For this review, take the finished solid that the model builds, in its own axes (mm). Coordinates: 2 decimals unless noted, no trailing zeros. Loops run counter-clockwise (first coordinate to the right, second up) from the corner with the lowest first, then second, coordinate; pieces in that order, holes last. Notation, with made-up numbers: (73, -30) - (104, -30) arc R16 ccw to (104, -22) - close; hole circle Ø10 at (43.25, 86). An arc over 180 degrees is marked (long way). Use one line per item in the form item = value. Start each with the question number.
1. For pin 1 Ø2 at (x, y) = (18, 4.5) entering from +Z, flat-tipped, find the tip position at first contact; note if it passes through.
2. Add section A-A on x = 0. Give the boundary of the cut face in (y, z), and give its area (3 significant figures).
3. Add section B-B on z = 0. Give the boundary of the cut face in (x, y), and give its area (3 significant figures).
4. To check wall thickness, follow probe 1 along Z at (x, y) = (0, 1.75); probe 2 along Z at (x, y) = (7, 0.75); probe 3 along X at (y, z) = (2.75, -31.5). State the ranges of each line that lie inside material, in increasing order.
5. Add section D-D on x = -11.5. Give the boundary of the cut face in (y, z), and give its area (3 significant figures).
6. Add section C-C on y = 4.25. Give the boundary of the cut face in (x, z) (1 decimal), and give its area (3 significant figures).
7. Draft analysis for pull direction Z (two halves, no side actions). For faces 1 (the face through (0.414, 3.131, 21.586)), 2 (the face through (3.097, 3.131, -24.152)), 3 (the face through (0, 0, -22)), 4 (the face through (14.274, 3.131, -0.628)), state which applies: +Z half, -Z half, draft (parallel to the pull), parting line (faces both ways), or undercut.
Autodesk Inventor part; units mm, degrees
ref_plane "YZ Plane" through (0, 0, 0) normal (1, 0, 0) x (0, 1, 0)
ref_plane "XZ Plane" through (0, 0, 0) normal (0, 1, 0) x (-1, 0, 0)
ref_plane "XY Plane" through (0, 0, 0) normal (0, 0, 1) x (1, 0, 0)
sketch "Sketch1" plane through (0, 0, 0) normal (0, 1, 0) x (-1, 0, 0)
  circle A0 centre (0, 0) radius 15.24 construction
  circle A1 centre (0, -38.1) radius 22.86 construction
  circle A2 centre (0, 0) radius 14.2875
  circle A3 centre (0, -38.1) radius 14.2875
  line L0 (-14.9321, 3.048) -> (-22.3981, -33.528) construction
  line L1 (14.9321, 3.048) -> (22.3981, -33.528) construction
  arc A4 (-22.3981, -33.528) -> (22.3981, -33.528) centre (0, -38.1) ccw construction
  arc A5 (14.9321, 3.048) -> (-14.9321, 3.048) centre (0, 0) ccw construction
  line L2 (28.6198, -32.258) -> (21.1538, 4.318)
  arc A6 (21.1538, 4.318) -> (-21.1538, 4.318) centre (0, 0) ccw
  line L3 (-21.1538, 4.318) -> (-28.6198, -32.258)
  arc A7 (-28.6198, -32.258) -> (28.6198, -32.258) centre (0, -38.1) ccw
  dimension "d0" = 30.48
  dimension "d1" = 45.72
  dimension "d2" = 28.575
  dimension "d3" = 28.575
  dimension "d4" = 6.35
extrude "Extrusion1" add sketch "Sketch1" along normal blind 6.35
properties part number "DTraining2_001_E1Base"
Conclusion:
q1.pin_1 = 13.31
q2.outline = (0, -67.31) - (6.35, -67.31) - (6.35, -52.39) - (0, -52.39) - close; (0, -23.81) - (6.35, -23.81) - (6.35, -14.29) - (0, -14.29) - close; (0, 14.29) - (6.35, 14.29) - (6.35, 21.59) - (0, 21.59) - close
q2.area = 202 mm^2
q3.outline = (-22.04, 0) - (-14.29, 0) - (-14.29, 6.35) - (-22.04, 6.35) - close; (14.29, 0) - (22.04, 0) - (22.04, 6.35) - (14.29, 6.35) - close
q3.area = 98.4 mm^2
q4.probe_1 = -67.31 to -52.39, -23.81 to -14.29, 14.29 to 21.59
q4.probe_2 = -66.46 to -50.56, -25.64 to -12.46, 12.46 to 20.42
q4.probe_3 = -28.47 to -12.67, 12.67 to 28.47
q5.outline = (0, -64.95) - (6.35, -64.95) - (6.35, -46.58) - (0, -46.58) - close; (0, -29.62) - (6.35, -29.62) - (6.35, -8.48) - (0, -8.48) - close; (0, 8.48) - (6.35, 8.48) - (6.35, 18.27) - (0, 18.27) - close
q5.area = 313 mm^2
q6.outline = (-28.6, -32.3) arc R29.2 ccw (long way) to (28.6, -32.3) - (21.2, 4.3) arc R21.6 ccw to (-21.2, 4.3) - close; hole circle Ø28.6 at (0, -38.1); hole circle Ø28.6 at (0, 0)
q6.area = 2,760 mm^2
q7.face_1 = +Z half
q7.face_2 = undercut
q7.face_3 = draft
q7.face_4 = undercut
